Read the model definition and answer for the solid it produces. Units are mm, in the model's axes. Face numbers are marked on the shaded views. A direction names the side the tool comes from. Coordinates: 2 decimals unless noted, no trailing zeros. Loops run counter-clockwise (first coordinate to the right, second up) from the corner with the lowest first, then second, coordinate; pieces in that order, holes last. Notation, with made-up numbers: (-7, 63.5) -> (45, 63.5) arc R21 ccw to (45, 82.5) -> close; hole circle Ø9 at (-34, 71). An arc over 180 degrees is marked (long way). Answer in a Markdown table with one row per item.
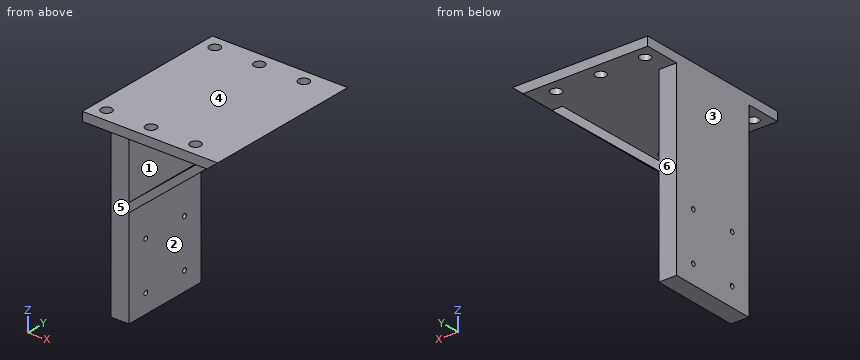
```python
from build123d import *

# Parameters (mm, degrees)
EXTRUDE_1_DEPTH     = 50
SKETCH_2_W          = 76
SKETCH_2_H          = 20
EXTRUDE_2_DEPTH     = 5
CUT_EXTRUDE_1_DEPTH = 44
SKETCH_5_R          = 1.25
CUT_EXTRUDE_2_DEPTH = 77
SKETCH_6_R          = 3
CUT_EXTRUDE_3_DEPTH = 6


with BuildPart() as part:
    # 草图1 → 凸台-拉伸1 (new body)
    with BuildSketch(Plane(origin=(0, 0, 0), x_dir=(1, 0, 0), z_dir=(0, 1, 0))):
        Polygon((0, 0), (0, 110), (10, 110), (10, 55), (76, 0), (70, 0), (10, 0), align=None)
        Polygon((64, 5), (10, 50), (10, 5), align=None, mode=Mode.SUBTRACT)
    extrude(amount=EXTRUDE_1_DEPTH)

    # 草图2 → 凸台-拉伸2 (add)
    with BuildSketch(Plane.XY):
        with Locations((38, 60)):
            Rectangle(SKETCH_2_W, SKETCH_2_H)
    extrude_2 = extrude(amount=-EXTRUDE_2_DEPTH)

    # 草图3 → 切除-拉伸1 (cut)
    with BuildSketch(Plane.XZ.offset(-50)):
        Polygon((70, -5), (76, 0), (76, -5), align=None)
    cut_extrude_1 = extrude(amount=-CUT_EXTRUDE_1_DEPTH, mode=Mode.SUBTRACT)

    # 镜向1: 凸台-拉伸2, 切除-拉伸1 across plane
    add(extrude_2.mirror(Plane(origin=(0, 25, 0), x_dir=(0, 0, 1), z_dir=(0, -1, 0))))
    add(cut_extrude_1.mirror(Plane(origin=(0, 25, 0), x_dir=(0, 0, 1), z_dir=(0, -1, 0))), mode=Mode.SUBTRACT)

    # 草图5 → 切除-拉伸2 (cut, through all)
    with BuildSketch(Plane.ZY):
        with Locations((-72.564971157, 38.435028843)):
            Circle(SKETCH_5_R)
        with Locations((-72.564971157, 11.564971157)):
            Circle(SKETCH_5_R)
        with Locations((-99.435028843, 11.564971157)):
            Circle(SKETCH_5_R)
        with Locations((-99.435028843, 38.435028843)):
            Circle(SKETCH_5_R)
    extrude(amount=-CUT_EXTRUDE_2_DEPTH, mode=Mode.SUBTRACT)

    # 草图6 → 切除-拉伸3 (cut, through all)
    with BuildSketch(Plane(origin=(0, 0, -5), x_dir=(-1, 0, 0), z_dir=(0, 0, -1))):
        with Locations((-7.5, 62.5)):
            Circle(SKETCH_6_R)
        with Locations((-32.5, 62.5)):
            Circle(SKETCH_6_R)
        with Locations((-57.5, 62.5)):
            Circle(SKETCH_6_R)
    cut_extrude_3 = extrude(amount=-CUT_EXTRUDE_3_DEPTH, mode=Mode.SUBTRACT)

    # 镜向2: 切除-拉伸3 across plane
    add(cut_extrude_3.mirror(Plane(origin=(0, 25, 0), x_dir=(0, 0, 1), z_dir=(0, -1, 0))), mode=Mode.SUBTRACT)


solid = part.part
```
1. A cutting plane is placed at C-C on y = 25.5. Give the vertices of the cut face in (x, z).
A:
| item | result |
|---|---|
| outline | (0, -110) -> (10, -110) -> (10, -55) -> (76, 0) -> (0, 0) -> close; hole (10, -50) -> (64, -5) -> (10, -5) -> close |
2. The mould has two halves that part along X. Classify the marked faces 1, 2, 3 and 4: pulls with the +X half, pulls with the -X half, needs draft (parallel to the pull), parting line crosses it, or undercut.
A:
| item | result |
|---|---|
| face 1 | undercut |
| face 2 | pulls with the +X half |
| face 3 | pulls with the -X half |
| face 4 | needs draft |
3. Given pin 1 Ø25 at (y, z) = (34.5, -92.5) entering from +X; pin 2 Ø1 at (y, z) = (2.5, -12) entering from +X; pin 3 Ø6 at (x, y) = (45.5, 57) entering from -Z, each flat-ended and moving along its own axis, determine where each tip first touches the part or whether it passes through.
A:
| item | result |
|---|---|
| pin 1 | stops at x = 10 |
| pin 2 | stops at x = 62.2 |
| pin 3 | stops at z = -5 |
4. A cutting plane is placed at A-A on x = 32.5. Give the vertices of the cut face in (y, z), and give its area (3 significant figures).
A:
| item | result |
|---|---|
| outline | (-20, -5) -> (-15.5, -5) -> (-15.5, 0) -> (-20, 0) -> close; (-9.5, -5) -> (59.5, -5) -> (59.5, 0) -> (-9.5, 0) -> close; (0, -36.25) -> (50, -36.25) -> (50, -31.25) -> (0, -31.25) -> close; (65.5, -5) -> (70, -5) -> (70, 0) -> (65.5, 0) -> close |
| area | 640 mm2 |
5. A tool of negligible diameter and unlimited length cuts with its end or side. For the marked faces 5 and 6, from which of +Z, -Z, +X, -X, +Y, -Y can it reach the whole face along a straight path? Write none if from no direction.
A:
| item | result |
|---|---|
| face 5 | -Z, +X, -X, -Y |
| face 6 | -Z, +X, -X, +Y |
6. Find the intervals of material crossed by probe 1 along Y at (x, z) = (57.5, -3.3); probe 2 along X at (y, z) = (-12, -2); probe 3 along X at (y, z) = (-12, -3), in increasing order.
A:
| item | result |
|---|---|
| probe 1 | y = -20 to -15.5, -9.5 to 59.5, 65.5 to 70 |
| probe 2 | x = 0 to 4.54, 10.46 to 29.54, 35.46 to 54.54, 60.46 to 73.6 |
| probe 3 | x = 0 to 4.54, 10.46 to 29.54, 35.46 to 54.54, 60.46 to 72.4 |
7. A cutting plane is placed at D-D on x = 7.5. Give the vertices of the cut face in (y, z).
A:
| item | result |
|---|---|
| outline | (-20, -5) -> (-15.5, -5) -> (-15.5, 0) -> (-20, 0) -> close; (-9.5, -5) -> (0, -5) -> (0, -110) -> (50, -110) -> (50, -5) -> (59.5, -5) -> (59.5, 0) -> (-9.5, 0) -> close; (65.5, -5) -> (70, -5) -> (70, 0) -> (65.5, 0) -> close; hole circle Ø2.5 at (11.56, -99.44); hole circle Ø2.5 at (11.56, -72.56); hole circle Ø2.5 at (38.44, -99.44); hole circle Ø2.5 at (38.44, -72.56) |
8. A cutting plane is placed at B-B on y = 62.5. Give the vertices of the cut face in (x, z).
A:
| item | result |
|---|---|
| outline | (0, -5) -> (4.5, -5) -> (4.5, 0) -> (0, 0) -> close; (10.5, -5) -> (29.5, -5) -> (29.5, 0) -> (10.5, 0) -> close; (35.5, -5) -> (54.5, -5) -> (54.5, 0) -> (35.5, 0) -> close; (60.5, -5) -> (70, -5) -> (76, 0) -> (60.5, 0) -> close |
